For this review, take the finished solid that the model builds, in its own axes (mm). A direction names the side the tool comes from. Coordinates: 2 decimals unless noted, no trailing zeros. Write each loop counter-clockwise with the first axis right and the second up, starting at its lowest first coordinate (ties: lowest second). Pieces come first, ordered by that corner, then holes.
```python
from build123d import *

# Parameters (mm, degrees)
F0_R     = 4
F0_W     = 20
F0_H     = 10
F1_DEPTH = 10
F2_R     = 4


with BuildPart() as f1:
    # F0 (on Top) → F1 (new body)
    with BuildSketch(Plane.XY):
        Polygon((10, 9), (15, 30), (10, 30), (-10, 30), (-15, 30), (-10, 9), (-10, 0), (-10, -9), (-15, -30), (-10, -30), (10, -30), (15, -30), (10, -9), (10, 0), align=None)
        Polygon((-5, -24), (0, -9), (5, -24), align=None, mode=Mode.SUBTRACT)
        Circle(F0_R, mode=Mode.SUBTRACT)
        Polygon((5, 24), (0, 9), (-5, 24), align=None, mode=Mode.SUBTRACT)
        with Locations((0, 35)):
            Rectangle(F0_W, F0_H)
        with Locations((0, -35)):
            Rectangle(F0_W, F0_H)
    extrude(amount=F1_DEPTH)

    # F2
    f2_edges = [f1.edges().sort_by_distance(p)[0] for p in [
        (-10, -35, 10),
        (10, -35, 10),
        (-10, -35, 0),
        (10, -35, 0),
        (10, 35, 0),
        (-10, 35, 0),
        (-10, 35, 10),
        (10, 35, 10),
    ]]
    fillet(f2_edges, radius=F2_R)


solid = f1.part
```
1) The part is to be moulded in two halves that separate along X. For faces 4 (the face through (8.859, -34.93, 8.797)), 5 (the face through (2.535, 16.605, 4.93)), 6 (the face through (13, 30, 5)), say which applies: pulls with the +X half, pulls with the -X half, needs draft (parallel to the pull), parting line crosses it, or undercut.
2) Consider section B-B (x = 1.25). Give the boundary of the cut face in (y, z), then the cut area to 3 significant figures.
3) Consider section C-C (y = -32.5). Give the boundary of the cut face in (x, z).
4) Clearance check with flat-ended pins moving along their axes: P1, Ø1.6, axis at y = -33, z = 5, coming from the -X side; P2, Ø4.5, axis at x = 12, z = 5, coming from the -Y side; P3, Ø3, axis at y = 26.5, z = 3, coming from the +X side; P4, Ø3, axis at y = 2.5, z = 4, coming from the +X side. State where each tip first meets the part, or that it passes through.
5) Consider section A-A (y = 0). Give the boundary of the cut face in (x, z).
6) Consider section D-D (y = -15.5). Give the boundary of the cut face in (x, z).
7) Tool access review of faces 1 (the face through (2.465, -16.395, 4.93)), 2 (the face through (10, 35, 5)), 3 (the face through (8.859, -34.93, 1.203)): name each direction out of +Z, -Z, +X, -X, +Y, -Y from which nothing blocks a thin tool from reaching the whole face with its end or side.
8) For L1, parallel to X at y = -5, z = 1.75; L2, parallel to X at y = -11, z = 8.75; L3, parallel to X at y = -10.5, z = 5.75, list the stretches that pass through material, from the lowest coordinate up.
Results:
1. face 4: pulls with the +X half
1. face 5: undercut
1. face 6: needs draft
2. outline: (-40, 0) - (-24, 0) - (-24, 10) - (-40, 10) - close; (-12.75, 0) - (-3.8, 0) - (-3.8, 10) - (-12.75, 10) - close; (3.8, 0) - (12.75, 0) - (12.75, 10) - (3.8, 10) - close; (24, 0) - (40, 0) - (40, 10) - (24, 10) - close
2. area: 499 mm2
3. outline: (-10, 4) arc R4 ccw to (-6, 0) - (6, 0) arc R4 ccw to (10, 4) - (10, 6) arc R4 ccw to (6, 10) - (-6, 10) arc R4 ccw to (-10, 6) - close
4. P1: stops at x = -10
4. P2: stops at y = -40
4. P3: stops at x = 14.52
4. P4: stops at x = 10
5. outline: (-10, 0) - (-4, 0) - (-4, 10) - (-10, 10) - close; (4, 0) - (10, 0) - (10, 10) - (4, 10) - close
6. outline: (-11.55, 0) - (-2.17, 0) - (-2.17, 10) - (-11.55, 10) - close; (2.17, 0) - (11.55, 0) - (11.55, 10) - (2.17, 10) - close
7. face 1: +Z, -Z
7. face 2: +Z, -Z, +X, +Y
7. face 3: -Z, +X, -Y
8. L1: x = -10 to 10
8. L2: x = -10.48 to -0.67, 0.67 to 10.48
8. L3: x = -10.36 to -0.5, 0.5 to 10.36
